Design review of the part built by this model. Coordinates are the model's own, in mm. Round coordinates to 2 decimals unless told otherwise and drop trailing zeros. Order: outer loops, then holes, each group sorted by start corner. A loop starts at its lowest first (then second) coordinate and runs counter-clockwise, first axis right, second up. Notation, with made-up numbers: M 80.5,44.5 L 136.5,44.5 A21 ccw 136.5,81.5 Z; hole C 64.25,-31 d3. An arc over 180 degrees is marked long. Use a Markdown table: item, result. Add a question column.
(1) Take a section at A-A (y = 10). Write out the cut boundary in (x, z).
(2) To check wall thickness, follow probe 1 along Y at (x, z) = (1, 3.5); probe 2 along X at (y, z) = (-8.5, 29.5); probe 3 along Z at (x, y) = (14.5, -1.5). State the ranges of each line that lie inside material, in increasing order. Write a range as from..to.
(3) Take a section at C-C (x = 0.5). Write out the cut boundary in (y, z), then the cut area to 3 significant figures.
(4) For pin 1 (12 mm diameter, centred on y = 1, z = 18.5, fed in from -X); pin 2 (1 mm diameter, centred on x = -8.5, y = 0.5, fed in from +Z); pin 3 (1.5 mm diameter, centred on x = -8, y = -8, fed in from +Z), all flat-tipped, find the tip position at first contact; note any pin that passes through.
(5) Take a section at D-D (y = 1). Write out the cut boundary in (x, z).
(6) Take a section at B-B (z = 7). Write out the cut boundary in (x, y), then the cut area to 3 significant figures.
```python
from build123d import *

# Parameters (mm, degrees)
F0_R     = 17.5
F1_DEPTH = 35
F3_DEPTH = 25


with BuildPart() as f1:
    # F0 (on Top) → F1 (new body)
    with BuildSketch(Plane.XY):
        Circle(F0_R)
    extrude(amount=F1_DEPTH)


with BuildPart() as f3:
    # F2 (on Front) → F3 (new body, symmetric)
    with BuildSketch(Plane.XZ):
        Polygon((0, 35), (-17.5, 0), (17.5, 0), align=None)
    extrude(amount=F3_DEPTH, both=True)


with BuildPart() as f1_1:
    add(f1.part)

    # F4: intersect F3
    add(f3.part, mode=Mode.INTERSECT)


solid = f1_1.part
```
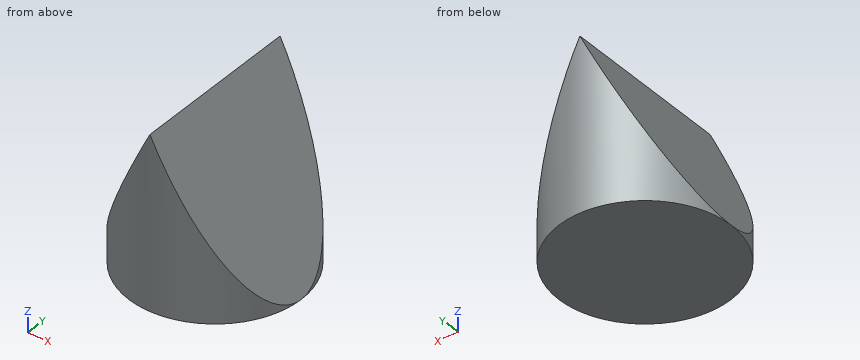
Verdict:
| question | item | result |
|---|---|---|
| 1 | outline | M -14.36,0 L 14.36,0 L 14.36,6.28 L 0,35 L -14.36,6.28 Z |
| 2 | probe 1 | y = -17.47..17.47 |
| 2 | probe 2 | x = -2.75..2.75 |
| 2 | probe 3 | z = 0..6 |
| 3 | outline | M -17.49,0 L 17.49,0 L 17.49,34 L -17.49,34 Z |
| 3 | area | 1,190 mm^2 |
| 4 | pin 1 | stops at x = -11.25 |
| 4 | pin 2 | stops at z = 19 |
| 4 | pin 3 | stops at z = 20.5 |
| 5 | outline | M -17.47,0 L 17.47,0 L 17.47,0.06 L 0,35 L -17.47,0.06 Z |
| 6 | outline | M -14,-10.5 A17.5 ccw 14,-10.5 L 14,10.5 A17.5 ccw -14,10.5 Z |
| 6 | area | 862 mm^2 |
